Can you work these out from the drawing? Everything is in mm from the part's minimum corner. A direction names the side the tool comes from. Give positions to 0.01 mm unless a question says otherwise; leave off trailing zeros. Loops run counter-clockwise (first coordinate to the right, second up) from the corner with the lowest first, then second, coordinate; pieces in that order, holes last. Notation, with made-up numbers: (-25.75, 0) -> (-10.75, 0) arc R21 cw to (-10.75, 4) -> close; hole circle Ø11 at (21.25, 31). An arc over 180 degrees is marked (long way). Return JSON: item names as keys, results as strings. Group by question number.
Q1. Suppose I cut it at C-C, the plane x = 34.5. Please give me the cut outline in (y, z).
Q2. Suppose I cut it at D-D, the plane z = 5. Please give me the cut outline in (x, y), and give its area (3 significant figures).
Q3. Thinking about a two-plate mould opening in X: for the marked faces 1, 2 and 3, which applies, pulls with the +X half, pulls with the -X half, needs draft (parallel to the pull), parting line crosses it, or undercut?
Q4. Suppose I cut it at A-A, the plane z = 17.5. Please give me the cut outline in (x, y).
Q5. Which directions (+Z, -Z, +X, -X, +Y, -Y) give clear straight access to the entire face, cutting with the end or side of a thin tool? Please do the marked faces 4 and 5.
Q6. I need wall thicknesses on line 1 along Y through (x, z) = (6.5, 7.25); line 2 along Y through (x, z) = (36.5, 4.25); line 3 along X through (y, z) = (13, 17.5). Which ranges of each line are inside material? Lowest first, please. Write a range as [from, to].
Q7. Will these pins go through, and if not, where does the flat tip stop? pin 1 (2.5 mm diameter, centred on x = 34, y = 33.5, fed in from -Z); pin 2 (10 mm diameter, centred on x = 20.5, y = 17, fed in from +Z) (1 decimal).
Q8. Suppose I cut it at B-B, the plane y = 23. Please give me the cut outline in (x, z).
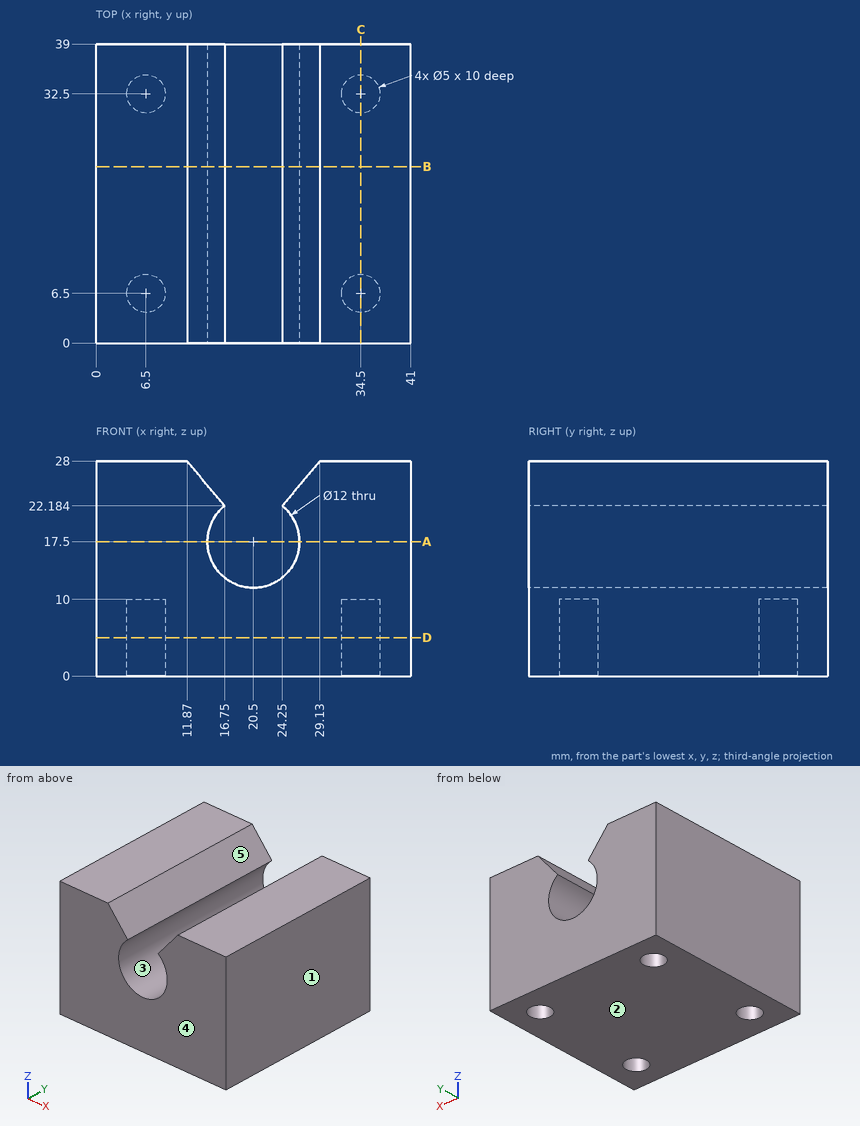
Ans:
{
 "1": {"outline": "(0, 0) -> (4, 0) -> (4, 10) -> (9, 10) -> (9, 0) -> (30, 0) -> (30, 10) -> (35, 10) -> (35, 0) -> (39, 0) -> (39, 28) -> (0, 28) -> close"},
 "2": {"outline": "(0, 0) -> (41, 0) -> (41, 39) -> (0, 39) -> close; hole circle Ø5 at (6.5, 6.5); hole circle Ø5 at (6.5, 32.5); hole circle Ø5 at (34.5, 6.5); hole circle Ø5 at (34.5, 32.5)", "area": "1,520 mm^2"},
 "3": {"face 1": "pulls with the +X half", "face 2": "needs draft", "face 3": "undercut"},
 "4": {"outline": "(0, 0) -> (14.5, 0) -> (14.5, 39) -> (0, 39) -> close; (26.5, 0) -> (41, 0) -> (41, 39) -> (26.5, 39) -> close"},
 "5": {"face 4": "+Z, -Z, +X, -X, -Y", "face 5": "+Z, +Y, -Y"},
 "6": {"line 1": "y = [0, 4], [9, 30], [35, 39]", "line 2": "y = [0, 5], [8, 31], [34, 39]", "line 3": "x = [0, 14.5], [26.5, 41]"},
 "7": {"pin 1": "stops at z = 10", "pin 2": "stops at z = 23.7"},
 "8": {"outline": "(0, 0) -> (41, 0) -> (41, 28) -> (29.13, 28) -> (24.25, 22.18) arc R6 cw (long way) to (16.75, 22.18) -> (11.87, 28) -> (0, 28) -> close"}
}
